```python
from build123d import *

# Parameters (mm, degrees)
SKETCH_W  = 65.75
SKETCH_H  = 46.5
PAD_DEPTH = 2.5


with BuildPart() as part:
    # Sketch → Pad (new body)
    with BuildSketch(Plane.XY):
        Rectangle(SKETCH_W, SKETCH_H)
        Polygon((-22.875, 13.25), (-17.875, 13.25), (-17.875, 13.75), (17.875, 13.75), (17.875, 13.25), (22.875, 13.25), (22.875, -13.25), (17.875, -13.25), (17.875, -13.75), (-17.875, -13.75), (-17.875, -13.25), (-22.875, -13.25), align=None, mode=Mode.SUBTRACT)
    extrude(amount=PAD_DEPTH)


solid = part.part
```
Verification items for the finished model (mm, model axes). A direction names the side the tool comes from. Give positions to 0.01 mm unless a question says otherwise; leave off trailing zeros. Order: outer loops, then holes, each group sorted by start corner. A loop starts at its lowest first (then second) coordinate and runs counter-clockwise, first axis right, second up. Notation, with made-up numbers: (-10, 58.25) -> (-4, 58.25) arc R7 ccw to (-4, 71.25) -> close; hole circle Ø8 at (49, 80.25). An arc over 180 degrees is marked (long way). Use a Markdown table: item, result.
1) Material ranges on probe 1 along X at (y, z) = (-8, 2.1) (3 decimals); probe 2 along Y at (x, z) = (-0.5, 0.4); probe 3 along Y at (x, z) = (-22, 1.9), recorded low to high.
Results:
| item | result |
|---|---|
| probe 1 | -32.875 to -22.875, 22.875 to 32.875 |
| probe 2 | -23.25 to -13.75, 13.75 to 23.25 |
| probe 3 | -23.25 to -13.25, 13.25 to 23.25 |
2) Section check B-B, the plane x = -2.5. Record the boundary of the cut face in (y, z), then the cut area to 3 significant figures.
Results:
| item | result |
|---|---|
| outline | (-23.25, 0) -> (-13.75, 0) -> (-13.75, 2.5) -> (-23.25, 2.5) -> close; (13.75, 0) -> (23.25, 0) -> (23.25, 2.5) -> (13.75, 2.5) -> close |
| area | 47.5 mm² |
3) Section check C-C, the plane z = 0.8. Record the boundary of the cut face in (x, y) (3 decimals), then the cut area to 3 significant figures.
Results:
| item | result |
|---|---|
| outline | (-32.875, -23.25) -> (32.875, -23.25) -> (32.875, 23.25) -> (-32.875, 23.25) -> close; hole (-22.875, -13.25) -> (-17.875, -13.25) -> (-17.875, -13.75) -> (17.875, -13.75) -> (17.875, -13.25) -> (22.875, -13.25) -> (22.875, 13.25) -> (17.875, 13.25) -> (17.875, 13.75) -> (-17.875, 13.75) -> (-17.875, 13.25) -> (-22.875, 13.25) -> close |
| area | 1,810 mm² |
4) Mould release check, pull along X, two halves, no side actions. Record for faces 1 (the flat face through (0, -23.25, 1)), 2 (the flat face through (-20, -13.25, 1)), 3 (the flat face through (-20, 13.25, 1)), 4 (the flat face through (-32.875, 0, 1)): pulls with the +X half, pulls with the -X half, needs draft (parallel to the pull), parting line crosses it, or undercut.
Results:
| item | result |
|---|---|
| face 1 | needs draft |
| face 2 | undercut |
| face 3 | undercut |
| face 4 | pulls with the -X half |
5) Depth check by flat-ended pin: pin 1 Ø6 at (x, y) = (-19, 6.5) entering from -Z. Enter the tip coordinate at first touch or a pass-through.
Results:
| item | result |
|---|---|
| pin 1 | through |
6) Section check A-A, the plane y = 0. Record the boundary of the cut face in (x, z) (3 decimals), then the cut area to 3 significant figures.
Results:
| item | result |
|---|---|
| outline | (-32.875, 0) -> (-22.875, 0) -> (-22.875, 2.5) -> (-32.875, 2.5) -> close; (22.875, 0) -> (32.875, 0) -> (32.875, 2.5) -> (22.875, 2.5) -> close |
| area | 50.0 mm² |
7) Tool access check on faces 5 (the flat face through (0, 23.25, 1)), 6 (the flat face through (22.875, 0, 1)). Record the directions out of +Z, -Z, +X, -X, +Y, -Y that give a thin tool (end or side, any length) a straight path to the whole face; none if there is none.
Results:
| item | result |
|---|---|
| face 5 | +Z, -Z, +X, -X, +Y |
| face 6 | +Z, -Z |
